Part print with two shaded views. Sizes in mm from the minimum x, y, z corner. A direction names the side the tool comes from. Give positions to 0.01 mm unless a question says otherwise; leave off trailing zeros. Order: outer loops, then holes, each group sorted by start corner. A loop starts at its lowest first (then second) coordinate and runs counter-clockwise, first axis right, second up. Notation, with made-up numbers: (72.25, 58.5) -> (81.25, 58.5) arc R33 cw to (81.25, 97.5) -> close; hole circle Ø6 at (-35, 76.25). An arc over 180 degrees is marked (long way). Write item = value, one per line. Start each with the question number.
Item 1: Band-saw the part on B-B on z = 4.05. Write the cut outline in (x, y) (3 decimals).
Item 2: Pull direction Y, two halves, no side cores. Call the marked faces 5, 6, 7 and 8: +Y half, -Y half, draft (parallel to the pull), parting line (faces both ways), or undercut.
Item 3: Drill centre lines: line 1 along X through (y, z) = (3.5, 4) (3 decimals); line 2 along X through (y, z) = (0.75, 2.75) (3 decimals); line 3 along Y through (x, z) = (2.5, 4). Where is each one in solid material? Low to high.
Item 4: Band-saw the part on D-D on y = 2.75. Write the cut outline in (x, z) (1 decimal).
Item 5: Band-saw the part on A-A on x = 7.5. Write the cut outline in (y, z) (3 decimals).
Item 6: Tool access for the marked faces 1, 2, 3 and 4: list every direction of +Z, -Z, +X, -X, +Y, -Y with a clear straight run to the whole face (end or side of a thin tool).
Item 7: Flat gauge pins, fed straight in: P1, Ø0.8, axis at x = 11, y = 11, coming from the +Z side; P2, Ø2, axis at y = 10.5, z = 4, coming from the -X side; P3, Ø3.5, axis at y = 3, z = 3, coming from the -X side (3 decimals); P4, Ø5, axis at x = 11, y = 5, coming from the -Z side. Where does each tip first touch, or does it go through?
Item 8: Band-saw the part on C-C on y = 12. Write the cut outline in (x, z) (3 decimals).
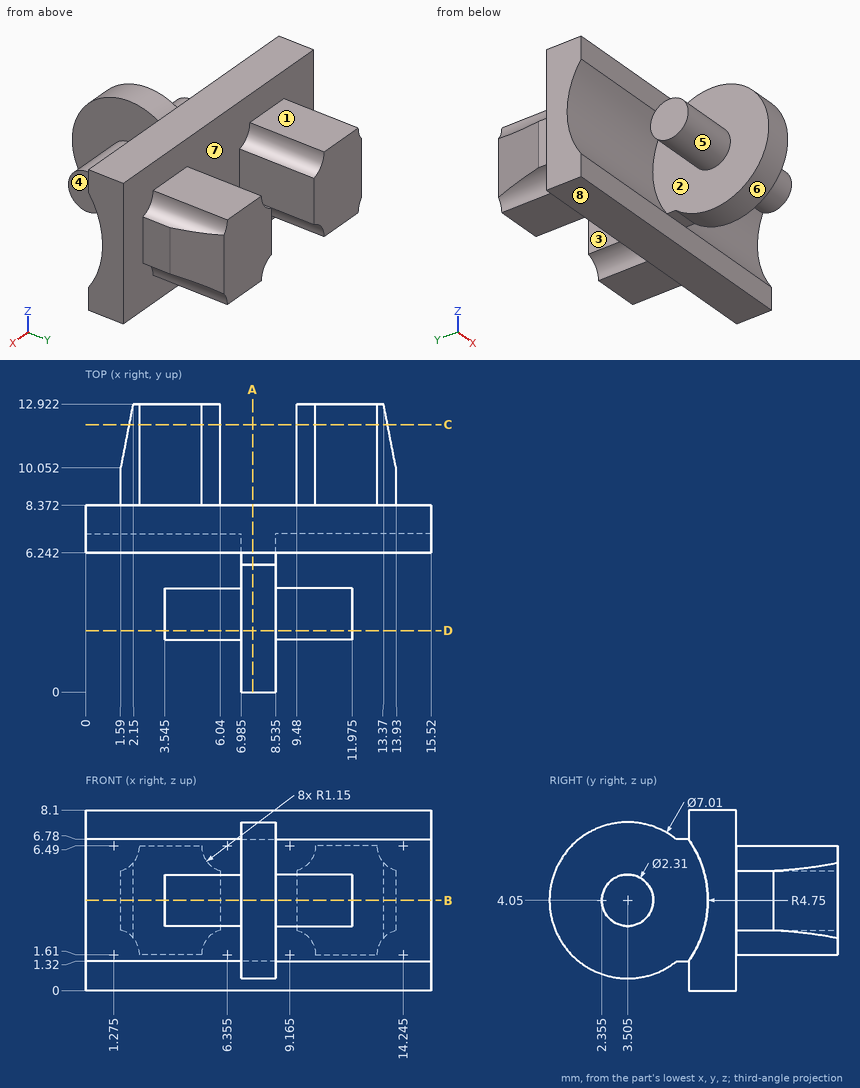
Values found:
q1.outline = (0, 7.105) -> (6.985, 7.105) -> (6.985, 4.66) -> (3.545, 4.66) -> (3.545, 2.35) -> (6.985, 2.35) -> (6.985, 0) -> (8.535, 0) -> (8.535, 2.35) -> (11.975, 2.35) -> (11.975, 4.66) -> (8.535, 4.66) -> (8.535, 7.105) -> (15.52, 7.105) -> (15.52, 8.372) -> (13.93, 8.372) -> (13.93, 10.052) -> (13.37, 12.922) -> (9.48, 12.922) -> (9.48, 8.372) -> (6.04, 8.372) -> (6.04, 12.922) -> (2.15, 12.922) -> (1.59, 10.052) -> (1.59, 8.372) -> (0, 8.372) -> close
q2.face_5 = undercut
q2.face_6 = undercut
q2.face_7 = +Y half
q2.face_8 = draft
q3.line_1 = 3.545 to 11.975
q3.line_2 = 6.985 to 8.535
q3.line_3 = 7.1 to 12.92
q4.outline = (3.5, 3.2) -> (7, 3.2) -> (7, 0.6) -> (8.5, 0.6) -> (8.5, 3.2) -> (12, 3.2) -> (12, 4.9) -> (8.5, 4.9) -> (8.5, 7.5) -> (7, 7.5) -> (7, 4.9) -> (3.5, 4.9) -> close
q5.outline = (5.703, 1.32) -> (6.242, 1.32) -> (6.242, 0) -> (8.372, 0) -> (8.372, 8.1) -> (6.242, 8.1) -> (6.242, 6.78) -> (5.703, 6.78) arc R3.505 ccw (long way) to start
q6.face_1 = +Z, +X, -X, +Y
q6.face_2 = -X
q6.face_3 = +Z, -Z, +Y
q6.face_4 = +Z, -Z, +X, -Y
q7.P1 = 6.49
q7.P2 = 1.59
q7.P3 = 3.545
q7.P4 = 0
q8.outline = (1.97, 2.526) arc R1.15 cw to (2.425, 1.61) -> (5.205, 1.61) arc R1.15 cw to (6.04, 2.716) -> (6.04, 5.384) arc R1.15 cw to (5.205, 6.49) -> (2.425, 6.49) arc R1.15 cw to (1.97, 5.574) -> close; (9.48, 2.716) arc R1.15 cw to (10.315, 1.61) -> (13.095, 1.61) arc R1.15 cw to (13.55, 2.526) -> (13.55, 5.574) arc R1.15 cw to (13.095, 6.49) -> (10.315, 6.49) arc R1.15 cw to (9.48, 5.384) -> close
